Drawing for the job (mm, zero at the part's lowest x, y, z). A direction names the side the tool comes from. Give positions to 0.01 mm unless a question says otherwise; leave off trailing zeros. Order: outer loops, then holes, each group sorted by start corner. A loop starts at its lowest first (then second) coordinate and runs counter-clockwise, first axis right, second up. Notation, with made-up numbers: M -21.75,-8 L 10.25,-8 A4 cw 10.25,-4 Z; hole C 77.25,-4.5 d3. An arc over 180 degrees is marked long. One line per item, written item: value.
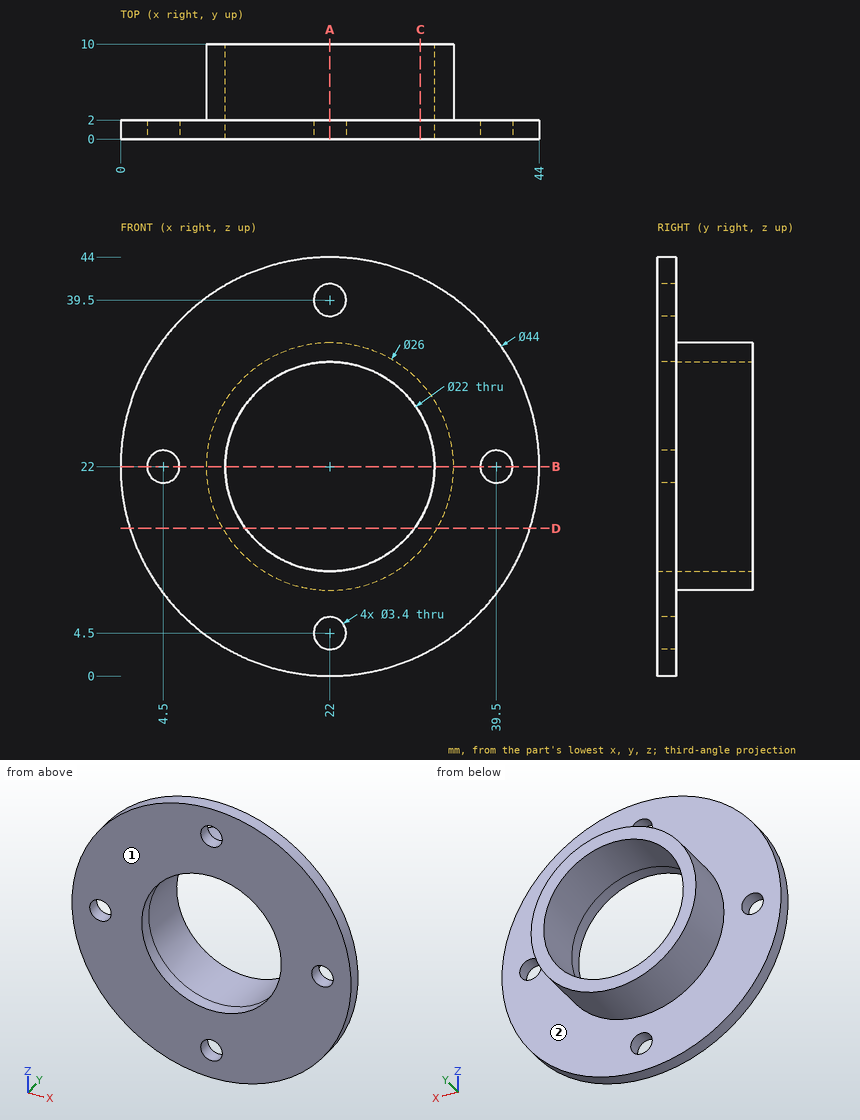
1) Tool access for the marked faces 1 and 2: list every direction of +Z, -Z, +X, -X, +Y, -Y with a clear straight run to the whole face (end or side of a thin tool).
Check values:
face 1: +Z, -Z, +X, -X, -Y
face 2: +Y
2) Pin check, flat tips, straight feed: pin 1 (2.5 mm diameter, centred on x = 4.5, z = 22, fed in from -Y); pin 2 (2 mm diameter, centred on x = 9.5, z = 10, fed in from +Y); pin 3 (1.5 mm diameter, centred on y = 6.5, z = 27, fed in from -X); pin 4 (5 mm diameter, centred on x = 18, y = 6.5, fed in from +Z). Stop position of each tip, or through.
Check values:
pin 1: through
pin 2: y = 2
pin 3: x = 9.71
pin 4: z = 34.91
3) Saw through at D-D, the plane z = 15.5. Write the cut outline in (x, y), then the cut area to 3 significant figures.
Check values:
outline: M 0.98,0 L 13.13,0 L 13.13,10 L 10.74,10 L 10.74,2 L 0.98,2 Z; M 30.87,0 L 43.02,0 L 43.02,2 L 33.26,2 L 33.26,10 L 30.87,10 Z
area: 86.7 mm^2
4) Saw through at C-C, the plane x = 31.5. Write the cut outline in (y, z), then the cut area to 3 significant figures.
Check values:
outline: M 0,2.16 L 2,2.16 L 2,13.13 L 10,13.13 L 10,16.45 L 0,16.45 Z; M 0,27.55 L 10,27.55 L 10,30.87 L 2,30.87 L 2,41.84 L 0,41.84 Z
area: 110 mm^2
5) Drill centre lines: probe 1 along X at (y, z) = (0.6, 22); probe 2 along Z at (x, y) = (22, 7.5). Where is each one in solid material? Low to high. Write a range as from..to.
Check values:
probe 1: 0..2.8, 6.2..11, 33..37.8, 41.2..44
probe 2: 9..11, 33..35
6) Saw through at B-B, the plane z = 22. Write the cut outline in (x, y).
Check values:
outline: M 0,0 L 2.8,0 L 2.8,2 L 0,2 Z; M 6.2,0 L 11,0 L 11,10 L 9,10 L 9,2 L 6.2,2 Z; M 33,0 L 37.8,0 L 37.8,2 L 35,2 L 35,10 L 33,10 Z; M 41.2,0 L 44,0 L 44,2 L 41.2,2 Z
7) Saw through at A-A, the plane x = 22. Write the cut outline in (y, z).
Check values:
outline: M 0,0 L 2,0 L 2,2.8 L 0,2.8 Z; M 0,6.2 L 2,6.2 L 2,9 L 10,9 L 10,11 L 0,11 Z; M 0,33 L 10,33 L 10,35 L 2,35 L 2,37.8 L 0,37.8 Z; M 0,41.2 L 2,41.2 L 2,44 L 0,44 Z
